Autodesk Inventor part; units mm, degrees
ref_plane "YZ Plane" through (0, 0, 0) normal (1, 0, 0) x (0, 1, 0)
ref_plane "XZ Plane" through (0, 0, 0) normal (0, 1, 0) x (-1, 0, 0)
ref_plane "XY Plane" through (0, 0, 0) normal (0, 0, 1) x (1, 0, 0)
sketch "Sketch1" plane through (0, 0, 0) normal (0, 0, 1) x (1, 0, 0)
  line L0 (4, 53.5) -> (4, 0)
  line L1 (4, 0) -> (24.75, 0)
  line L2 (24.75, 0) -> (24.75, 55.5)
  line L3 (24.75, 55.5) -> (0, 55.5)
  line L4 (24.75, 13) -> (24.75, 12)
  line L5 (24.75, 12) -> (15.6045, 12)
  line L6 (15.6045, 12) -> (15.6045, 13)
  line L7 (15.6045, 13) -> (24.75, 13)
  line L8 (24.75, 13) -> (24.75, 12)
  line L9 (4, 53.5) -> (8.87, 53.5)
  line L10 (8.87, 53.5) -> (8.87, 55.5)
  line L11 (0, 55.5) -> (0, 0)
  point P0 (8.87, 54.5)
  dimension "d2" = 55.5
  dimension "d32" = 1
  dimension "d33" = 12
  dimension "d36" = 2
  dimension "d37" = 49.5
  dimension "d38" = 8
  dimension "d39" = 17.74
revolve "Revolution1" add sketch "Sketch1" angle 360 about axis through (0, 55.5, 0) along (0, -1, 0)
sketch "Sketch2" plane through (0, 0, 0) normal (0, -1, 0) x (1, 0, 0)
  circle A0 centre (19, 0) radius 2
  circle A1 centre (0, 0) radius 4 construction
  line L0 (0, 0) -> (19, 0) construction
  circle A2 centre (0, 19) radius 2
  circle A3 centre (-19, 0) radius 2
  circle A4 centre (0, -19) radius 2
  point P0 (0, 0)
  dimension "d5" = 4
  dimension "d6" = 19
  dimension "d9" = 360
extrude "Extrusion1" cut sketch "Sketch2" against normal blind 5
chamfer "Chamfer1" distance 1.6 angle 45 1 edges at (-24.75, 55.5, 0)
chamfer "Chamfer2" distance 2.5 distance2 10 1 edges at (-24.75, 0, 0) measured on face at (13.1279, 0, -6.9036)
properties part number "5065"
CAD build for the part. Positions are in the model's coordinates, mm. A direction names the side the tool comes from. Give positions to 0.01 mm unless a question says otherwise; leave off trailing zeros. Write each loop counter-clockwise with the first axis right and the second up, starting at its lowest first coordinate (ties: lowest second). Pieces come first, ordered by that corner, then holes. Notation, with made-up numbers: (10.5, 23) -> (51.5, 23) arc R21 cw to (51.5, 43) -> close; hole circle Ø4 at (-19.5, 58). An arc over 180 degrees is marked (long way). Return JSON: item names as keys, results as strings.
Item 1: Drop flat-ended pins along their axis: pin 1 (6.5 mm diameter, centred on x = 0, z = 0, fed in from +Y); pin 2 (3 mm diameter, centred on x = -8, y = 12, fed in from +Z); pin 3 (1.5 mm diameter, centred on x = 2, y = 45, fed in from +Z); pin 4 (3 mm diameter, centred on x = -19, z = 0, fed in from -Y). Give the stop position or say it passes through.
Answer below:
{"pin 1": "passes through", "pin 2": "stops at z = 23.88", "pin 3": "stops at z = 24.72", "pin 4": "stops at y = 5"}
Item 2: Drill centre lines: probe 1 along Z at (x, y) = (0, 10.5); probe 2 along Z at (x, y) = (0, 3); probe 3 along Z at (x, y) = (1, 22.5). Where is each one in solid material? Low to high.
Answer below:
{"probe 1": "z = -24.75 to -4, 4 to 24.75", "probe 2": "z = -23 to -21, -17 to -4, 4 to 17, 21 to 23", "probe 3": "z = -24.73 to -3.87, 3.87 to 24.73"}
Item 3: Band-saw the part on A-A (z = 0). List the corners of the cut face in (x, y).
Answer below:
{"outline": "(-24.75, 10) -> (-22.25, 0) -> (-21, 0) -> (-21, 5) -> (-17, 5) -> (-17, 0) -> (-4, 0) -> (-4, 53.5) -> (-8.87, 53.5) -> (-8.87, 55.5) -> (-23.15, 55.5) -> (-24.75, 53.9) -> close; (4, 0) -> (17, 0) -> (17, 5) -> (21, 5) -> (21, 0) -> (22.25, 0) -> (24.75, 10) -> (24.75, 53.9) -> (23.15, 55.5) -> (8.87, 55.5) -> (8.87, 53.5) -> (4, 53.5) -> close"}
Item 4: Band-saw the part on B-B (y = 39). List the corners of the cut face in (x, z).
Answer below:
{"outline": "circle Ø49.5 at (0, 0); hole circle Ø8 at (0, 0)"}
Item 5: Two-plate mould, pull along Z, no slides. Class faces 1 (the flat face through (0, 5, -19)), 2 (the flat face through (0, 0, -5)), 3 (the conical face through (12.05, 0.63, -18.89)): +Z half, -Z half, draft (parallel to the pull), parting line (faces both ways), or undercut.
Answer below:
{"face 1": "undercut", "face 2": "draft", "face 3": "parting line"}
Item 6: Tool access for faces 4 (the flat face through (10, 55.5, 0)), 5 (the flat face through (19, 5, 0)), 6 (the cylindrical face through (4.09, 54.51, 7.87)): list every direction of +Z, -Z, +X, -X, +Y, -Y with a clear straight run to the whole face (end or side of a thin tool).
Answer below:
{"face 4": "+Z, -Z, +X, -X, +Y", "face 5": "-Y", "face 6": "+Y"}
